Design review of the part built by this model. Coordinates are the model's own, in mm. Give positions to 0.01 mm unless a question says otherwise; leave off trailing zeros. Loops run counter-clockwise (first coordinate to the right, second up) from the corner with the lowest first, then second, coordinate; pieces in that order, holes last.
Autodesk Fusion 360 part; units mm, degrees
sketch "Sketch1" plane through (0, 0, 0) normal (0, 0, 1) x (1, 0, 0)
  line L0 (54.5, -188.5) -> (-54.5, -188.5)
  line L1 (-54.5, -188.5) -> (-54.5, 188.5)
  line L2 (-54.5, 188.5) -> (54.5, 188.5)
  line L3 (54.5, 188.5) -> (54.5, -188.5)
  line L4 (54.5, -188.5) -> (-54.5, 188.5) construction
  line L5 (-54.5, -188.5) -> (54.5, 188.5) construction
  line L6 (-54.5, 153.5) -> (-39.5, 153.5)
  line L7 (-39.5, 153.5) -> (-39.5, 83.5)
  line L8 (-39.5, 83.5) -> (-54.5, 83.5)
  line L9 (-54.5, 83.5) -> (-54.5, 153.5)
  line L10 (-54.5, -153.5) -> (-39.5, -153.5)
  line L11 (-39.5, -153.5) -> (-39.5, -83.5)
  line L12 (-39.5, -83.5) -> (-54.5, -83.5)
  line L13 (-54.5, -83.5) -> (-54.5, -153.5)
  line L14 (54.5, -153.5629) -> (39.5, -153.5629)
  line L15 (39.5, -153.5629) -> (39.5, -83.5629)
  line L16 (39.5, -83.5629) -> (54.5, -83.5629)
  line L17 (54.5, -83.5629) -> (54.5, -153.5629)
  line L18 (54.5, 153.5) -> (39.5, 153.5)
  line L19 (39.5, 153.5) -> (39.5, 83.5)
  line L20 (39.5, 83.5) -> (54.5, 83.5)
  line L21 (54.5, 83.5) -> (54.5, 153.5)
  line L22 (-39.5, 153.5) -> (-39.5, 168.5)
  line L23 (-39.5, 168.5) -> (39.5, 168.5)
  line L24 (39.5, 153.5) -> (39.5, 168.5)
  line L25 (-39.5, -153.5) -> (-39.5, -168.5)
  line L26 (-39.5, -168.5) -> (39.5, -168.5)
  line L27 (39.5, -168.5) -> (39.5, -153.5629)
  dimension "d1" = 109
  dimension "d2" = 377
  dimension "d3" = 15
  dimension "d4" = 70
  dimension "d5" = 15
  dimension "d6" = 70
  dimension "d7" = 35
  dimension "d8" = 35
  dimension "d9" = 15
  dimension "d10" = 70
  dimension "d11" = 15
  dimension "d12" = 70
  dimension "d19" = 15
  dimension "d20" = 15
extrude "Extrude1" add sketch "Sketch1" along normal blind 5 contours L1 L3 L7 L8 L11 L12 L15 L16 L19 L20 L22 L23 L24 L25 L26 L27
fillet "Fillet1" radius 10 8 edges at (-39.5, -83.5, 2.5) (-54.5, -83.5, 2.5) (39.5, -83.5629, 2.5) (54.5, -83.5629, 2.5) (39.5, 83.5, 2.5) (54.5, 83.5, 2.5) (-39.5, 83.5, 2.5) (-54.5, 83.5, 2.5)
fillet "Fillet2" radius 15 4 edges at (-39.5, -168.5, 2.5) (39.5, -168.5, 2.5) (39.5, 168.5, 2.5) (-39.5, 168.5, 2.5)
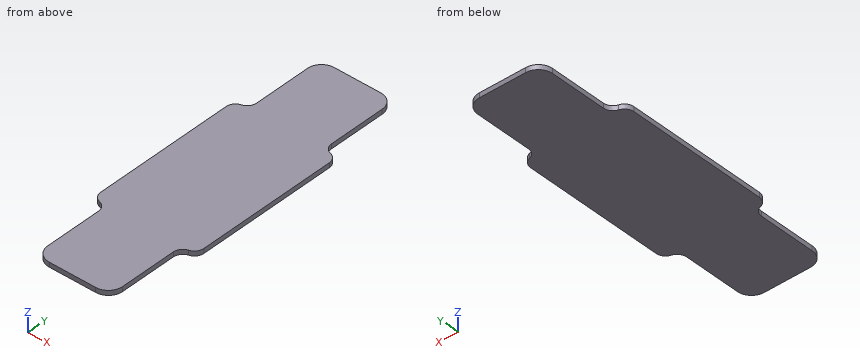
Q1. Insertion check: pin 1 (1.5 mm diameter, centred on y = -123.5, z = 2.5, fed in from -X). The pin has a flat end and moves straight along its axis. Give the tip position at first contact, or say it passes through.
Results:
pin 1: stops at x = -39.5
Q2. Wall thickness on line 1 (X direction, y = 75, z = 3.55); line 2 (X direction, y = -93.5, z = 3.15); line 3 (Y direction, x = -32, z = 0.55): over which ranges is each line inside the solid? List them lowest first.
Results:
line 1: x = -54.46 to 54.46
line 2: x = -39.5 to 39.5
line 3: y = -166.49 to 166.49
Q3. Take a section at A-A (y = -110.5). Give the boundary of the cut face in (x, z), plus the area to 3 significant figures.
Results:
outline: (-39.5, 0) - (39.5, 0) - (39.5, 5) - (-39.5, 5) - close
area: 395 mm2
Q4. Take a section at B-B (x = 34.5). Give the boundary of the cut face in (y, z), plus the area to 3 significant figures.
Results:
outline: (-164.68, 0) - (164.68, 0) - (164.68, 5) - (-164.68, 5) - close
area: 1,650 mm2
